Here's how the part is built. I have some questions about the finished solid (model axes, mm). A direction names the side the tool comes from. Round coordinates to 2 decimals unless told otherwise and drop trailing zeros. Loops run counter-clockwise (first coordinate to the right, second up) from the corner with the lowest first, then second, coordinate; pieces in that order, holes last. Notation, with made-up numbers: (73.5, 75.5) -> (122.5, 75.5) arc R15 ccw to (122.5, 84.5) -> close; hole circle Ø6 at (-22.5, -32). An arc over 180 degrees is marked (long way). Use CSV: the item, a comma, the result in double quotes. Start each with the question number.
from build123d import *

# Parameters (mm, degrees)
SKETCH_1_W          = 86
SKETCH_1_H          = 174
SKETCH_1_W_2        = 50
SKETCH_1_H_2        = 25
SKETCH_1_H_3        = 55
SKETCH_1_W_3        = 76
SKETCH_1_H_4        = 43
EXTRUDE_1_DEPTH     = 5
SKETCH_4_W          = 68.7
SKETCH_4_H          = 115
SKETCH_4_W_2        = 64.7
SKETCH_4_H_2        = 37
SKETCH_4_H_3        = 70
EXTRUDE_2_DEPTH     = 10
SKETCH_5_R          = 0.75
CUT_EXTRUDE_1_DEPTH = 122.783619588
SKETCH_7_W          = 15
SKETCH_7_H          = 8
SKETCH_7_W_2        = 26
SKETCH_7_W_3        = 5
SKETCH_7_H_2        = 10
SKETCH_7_H_3        = 12.119700025
SKETCH_7_W_4        = 6
SKETCH_7_H_4        = 5
SKETCH_7_W_5        = 7
SKETCH_7_H_5        = 21
CUT_EXTRUDE_2_DEPTH = 2
SKETCH_8_R          = 0.75
CUT_EXTRUDE_3_DEPTH = 2
CUT_EXTRUDE_START   = -84
SKETCH_8_3_R        = 0.75
CUT_EXTRUDE_4_DEPTH = 2


with BuildPart() as part:
    # 草图1 → 凸台-拉伸1 (new body)
    with BuildSketch(Plane(origin=(0, 0, 0), x_dir=(1, 0, 0), z_dir=(0, 1, 0))):
        with Locations((0, -26.5)):
            Rectangle(SKETCH_1_W, SKETCH_1_H)
        with Locations((0, -38)):
            Rectangle(SKETCH_1_W_2, SKETCH_1_H_2, mode=Mode.SUBTRACT)
        with Locations((0, 23)):
            Rectangle(SKETCH_1_W_2, SKETCH_1_H_3, mode=Mode.SUBTRACT)
        with Locations((0, -87)):
            Rectangle(SKETCH_1_W_3, SKETCH_1_H_4, mode=Mode.SUBTRACT)
    extrude(amount=EXTRUDE_1_DEPTH)

    # 草图4 → 凸台-拉伸2 (add)
    with BuildSketch(Plane(origin=(0, 5, 0), x_dir=(1, 0, 0), z_dir=(0, 1, 0))):
        Rectangle(SKETCH_4_W, SKETCH_4_H)
        with Locations((0, -37)):
            Rectangle(SKETCH_4_W_2, SKETCH_4_H_2, mode=Mode.SUBTRACT)
        with Locations((0, 20.5)):
            Rectangle(SKETCH_4_W_2, SKETCH_4_H_3, mode=Mode.SUBTRACT)
    extrude(amount=EXTRUDE_2_DEPTH)

    # 草图5 → 切除-拉伸1 (cut, through all)
    with BuildSketch(Plane(origin=(0, 5, 0), x_dir=(1, 0, 0), z_dir=(0, 1, 0))):
        with Locations(Location((-39, 20.5, 0), (0, 0, 270))):
            Circle(SKETCH_5_R)
        with Locations(Location((39, 20.5, 0), (0, 0, 270))):
            Circle(SKETCH_5_R)
        with Locations(Location((-39, -32.5, 0), (0, 0, 270))):
            Circle(SKETCH_5_R)
        with Locations(Location((39, -32.5, 0), (0, 0, 270))):
            Circle(SKETCH_5_R)
        with Locations(Location((-40.1427775, -60.35, 0), (0, 0, 270))):
            Circle(SKETCH_5_R)
        with Locations(Location((40.1427775, -60.35, 0), (0, 0, 270))):
            Circle(SKETCH_5_R)
        with Locations(Location((-40.1427775, -110.530299975, 0), (0, 0, 270))):
            Circle(SKETCH_5_R)
        with Locations(Location((40.1427775, -110.530299975, 0), (0, 0, 270))):
            Circle(SKETCH_5_R)
        with Locations(Location((-40.5, 57.5, 0), (0, 0, 270))):
            Circle(SKETCH_5_R)
        with Locations(Location((-40.5, -38, 0), (0, 0, 270))):
            Circle(SKETCH_5_R)
        with Locations(Location((-40.5, -85.5, 0), (0, 0, 270))):
            Circle(SKETCH_5_R)
        with Locations(Location((40.5, 57.5, 0), (0, 0, 270))):
            Circle(SKETCH_5_R)
        with Locations(Location((40.5, -38, 0), (0, 0, 270))):
            Circle(SKETCH_5_R)
        with Locations(Location((40.5, -85.5, 0), (0, 0, 270))):
            Circle(SKETCH_5_R)
        with Locations(Location((-40.5, -4.5, 0), (0, 0, 270))):
            Circle(SKETCH_5_R)
        with Locations(Location((40.5, -4.5, 0), (0, 0, 270))):
            Circle(SKETCH_5_R)
    extrude(amount=-CUT_EXTRUDE_1_DEPTH, mode=Mode.SUBTRACT)

    # 草图7 → 切除-拉伸2 (cut)
    with BuildSketch(Plane(origin=(0, 5, 0), x_dir=(1, 0, 0), z_dir=(0, 1, 0))):
        with Locations((-24.5, -61.5)):
            Rectangle(SKETCH_7_W, SKETCH_7_H)
        with Locations((0, -61.5)):
            Rectangle(SKETCH_7_W_2, SKETCH_7_H)
        with Locations((-40.5, -78.5)):
            Rectangle(SKETCH_7_W_3, SKETCH_7_H_2)
        with Locations((-40.5, -101.440149988)):
            Rectangle(SKETCH_7_W_3, SKETCH_7_H_3)
        with Locations((-32, -111)):
            Rectangle(SKETCH_7_W_4, SKETCH_7_H_4)
        with Locations((-3, -111)):
            Rectangle(SKETCH_7_W_4, SKETCH_7_H_4)
        with Locations((17.5, -111)):
            Rectangle(SKETCH_7_W_5, SKETCH_7_H_4)
        with Locations((30.5, -111)):
            Rectangle(SKETCH_7_W_5, SKETCH_7_H_4)
        with Locations((40.5, -92)):
            Rectangle(SKETCH_7_W_3, SKETCH_7_H_5)
    extrude(amount=-CUT_EXTRUDE_2_DEPTH, mode=Mode.SUBTRACT)

    # 草图8 → 切除-拉伸3 (cut)
    with BuildSketch(Plane.ZY.offset(43)):
        with Locations((8, 2.5)):
            Circle(SKETCH_8_R)
        with Locations((23, 2.5)):
            Circle(SKETCH_8_R)
        with Locations((52, 2.5)):
            Circle(SKETCH_8_R)
        with Locations((63, 2.5)):
            Circle(SKETCH_8_R)
    extrude(amount=-CUT_EXTRUDE_3_DEPTH, mode=Mode.SUBTRACT)

    # 草图8<3> → 切除-拉伸4 (cut)
    with BuildSketch(Plane.ZY.offset(43).offset(CUT_EXTRUDE_START)):
        with Locations((8, 2.5)):
            Circle(SKETCH_8_3_R)
        with Locations((23, 2.5)):
            Circle(SKETCH_8_3_R)
        with Locations((52, 2.5)):
            Circle(SKETCH_8_3_R)
        with Locations((63, 2.5)):
            Circle(SKETCH_8_3_R)
    extrude(amount=-CUT_EXTRUDE_4_DEPTH, mode=Mode.SUBTRACT)


solid = part.part
Q1. If we mould it in two halves opening along Z, with no side actions, what happens to faces 1 (the flat face through (34.35, 10, 1)), 2 (the flat face through (-41, 3, 78)), 3 (the flat face through (-38, 2, 87)), 4 (the flat face through (0, 10, -57.5))? For each: pulls with the +Z half, pulls with the -Z half, needs draft (parallel to the pull), parting line crosses it, or undercut.
Q2. I want a section at A-A, the plane x = 11. List the corners of the cut face in (y, z) for me.
Q3. Will these pins go through, and if not, where does the flat tip stop? pin 1 Ø1.5 at (x, y) = (18.5, 5) entering from +Z; pin 2 Ø0.8 at (y, z) = (2.5, 8) entering from -X; pin 3 Ø3 at (y, z) = (12, -9.5) entering from +X.
Q4. I want a section at B-B, the plane z = 79. List the corners of the cut face in (x, y) for me.
Q5. I need wall thicknesses on line 1 along Z through (x, y) = (-3.5, 5.75); line 2 along Z through (x, y) = (27, 2.5); line 3 along Z through (x, y) = (3, 4). Which ranges of each line are inside material? Lowest first, please.
Q6. I want a section at C-C, the plane y = 7.75. List the corners of the cut face in (x, z) for me.
Q7. For faces 5 (the flat face through (28, 5, -21)), 6 (the flat face through (0, 2, -50.5)), 7 (the flat face through (30, 3, 111)), which set-ups out of +Z, -Z, +X, -X, +Y, -Y let a thin tool reach every point of the face, with its end or its side?
Values found:
1,face 1,"needs draft"
1,face 2,"undercut"
1,face 3,"undercut"
1,face 4,"pulls with the -Z half"
2,outline,"(0, -60.5) -> (5, -60.5) -> (5, -57.5) -> (15, -57.5) -> (15, -55.5) -> (5, -55.5) -> (5, -50.5) -> (0, -50.5) -> close; (0, 4.5) -> (5, 4.5) -> (5, 14.5) -> (15, 14.5) -> (15, 18.5) -> (5, 18.5) -> (5, 25.5) -> (0, 25.5) -> close; (0, 50.5) -> (5, 50.5) -> (5, 55.5) -> (15, 55.5) -> (15, 57.5) -> (3, 57.5) -> (3, 65.5) -> (0, 65.5) -> close; (0, 108.5) -> (5, 108.5) -> (5, 113.5) -> (0, 113.5) -> close"
3,pin 1,"z = 65.5"
3,pin 2,"x = -41"
3,pin 3,"x = 34.35"
4,outline,"(-43, 0) -> (-38, 0) -> (-38, 3) -> (-43, 3) -> close; (38, 0) -> (43, 0) -> (43, 5) -> (38, 5) -> close"
5,line 1,"-57.5 to -55.5, 14.5 to 18.5, 55.5 to 57.5"
5,line 2,"-60.5 to 65.5, 108.5 to 113.5"
5,line 3,"-60.5 to -50.5, 4.5 to 25.5, 50.5 to 57.5, 108.5 to 113.5"
6,outline,"(-34.35, -57.5) -> (34.35, -57.5) -> (34.35, 57.5) -> (-34.35, 57.5) -> close; hole (-32.35, -55.5) -> (32.35, -55.5) -> (32.35, 14.5) -> (-32.35, 14.5) -> close; hole (-32.35, 18.5) -> (32.35, 18.5) -> (32.35, 55.5) -> (-32.35, 55.5) -> close"
7,face 5,"+Y"
7,face 6,"+Y, -Y"
7,face 7,"+Z, +Y"
